Answer from the drawing. Dimensions are ordinates in mm from the lowest x, y and z of the part. Give positions to 0.01 mm unless a question says otherwise; leave off trailing zeros. Order: outer loops, then holes, each group sorted by start corner. A loop starts at its lowest first (then second) coordinate and runs counter-clockwise, first axis right, second up. Notation, with made-up numbers: M 85,41 L 107,41 A33 cw 107,78 Z; hole C -21,47.5 d6. An arc over 180 degrees is marked long. One line per item, written item: value.
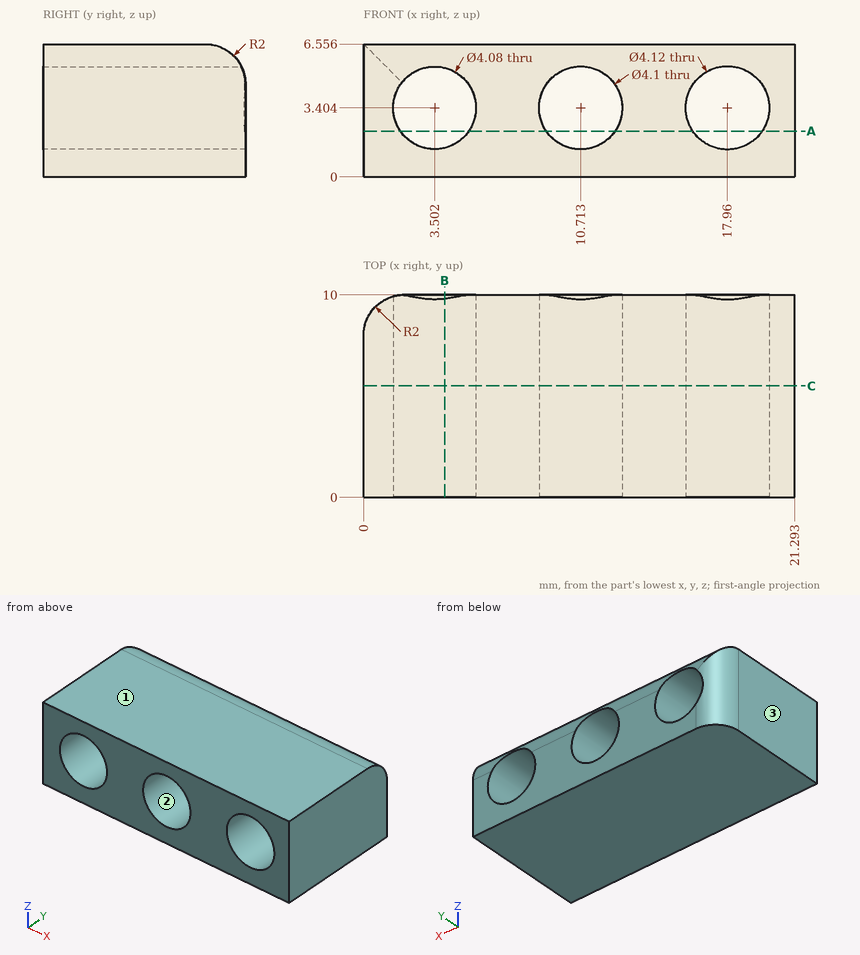
(1) Section A-A, the plane z = 2.25 is taken. Give the vertices of the cut face in (x, y) (1 decimal).
Findings:
outline: M 0,0 L 1.8,0 L 1.8,10 A2 ccw 0,8 Z; M 5.2,0 L 9,0 L 9,10 L 5.2,10 Z; M 12.4,0 L 16.3,0 L 16.3,10 L 12.4,10 Z; M 19.7,0 L 21.3,0 L 21.3,10 L 19.7,10 Z
(2) Determine the mould class of the marked faces 1, 2 and 3 for opening direction Z: pulls with the +Z half, pulls with the -Z half, needs draft (parallel to the pull), parting line crosses it, or undercut.
Findings:
face 1: pulls with the +Z half
face 2: undercut
face 3: needs draft
(3) Find the intervals of material crossed by probe 1 along X at (y, z) = (1.25, 3.25) (1 decimal); probe 2 along X at (y, z) = (3.75, 1.75) (1 decimal); probe 3 along Z at (x, y) = (10.5, 5.25) (1 decimal), in increasing order. Write a range as from..to.
Findings:
probe 1: x = 0..1.5, 5.5..8.7, 12.8..15.9, 20..21.3
probe 2: x = 0..2.3, 4.7..9.5, 11.9..16.7, 19.2..21.3
probe 3: z = 0..1.4, 5.4..6.6
(4) Section B-B, the plane x = 4 is taken. Give the vertices of the cut face in (y, z) (1 decimal).
Findings:
outline: M 0,0 L 10,0 L 10,1.4 L 0,1.4 Z; M 0,5.4 L 9.8,5.4 A2 ccw 8,6.6 L 0,6.6 Z
(5) Section C-C, the plane y = 5.5 is taken. Give the number of separate pieces and of enclosed holes in the cut face.
Findings:
separate pieces: 1
enclosed holes: 3
